from build123d import *

# Parameters (mm, degrees)
ESQUISSE1_W        = 58.2
ESQUISSE1_H        = 40
BOSS_EXTRU_1_DEPTH = 27
ESQUISSE2_R        = 15.5
BOSS_EXTRU_2_DEPTH = 57
ESQUISSE3_R        = 0.796993634
ESQUISSE3_R_2      = 3
ESQUISSE3_R_3      = 2.5
ESQUISSE3_R_4      = 1.643785586
BOSS_EXTRU_3_DEPTH = 1
ESQUISSE4_R        = 0.796993634
ESQUISSE4_R_2      = 3
ESQUISSE4_R_3      = 2.765269511
ESQUISSE4_R_4      = 2.5
ESQUISSE4_R_5      = 2.472480212
ESQUISSE4_R_6      = 1.643785586
BOSS_EXTRU_4_DEPTH = 1
ESQUISSE5_R        = 8.5
BOSS_EXTRU_5_DEPTH = 2
ESQUISSE6_R        = 3.91408695
BOSS_EXTRU_6_DEPTH = 13


with BuildPart() as part:
    # Esquisse1 → Boss.-Extru.1 (new body)
    with BuildSketch(Plane.XY):
        with Locations((-1.276315789, -5.258552632)):
            Rectangle(ESQUISSE1_W, ESQUISSE1_H)
    extrude(amount=BOSS_EXTRU_1_DEPTH)

    # Esquisse2 → Boss.-Extru.2 (add)
    with BuildSketch(Plane(origin=(27.823684211, 0, 0), x_dir=(0, 0, -1), z_dir=(1, 0, 0))):
        with Locations((-15.74475958, -4.690804329)):
            Circle(ESQUISSE2_R)
    extrude(amount=BOSS_EXTRU_2_DEPTH)

    # Esquisse3 → Boss.-Extru.3 (add)
    with BuildSketch(Plane(origin=(0, 0, 0), x_dir=(-1, 0, 0), z_dir=(0, 0, -1))):
        with Locations((28.393888361, 12.845029268)):
            Circle(ESQUISSE3_R)
        with Locations((28.393888361, -23.584885169)):
            Circle(ESQUISSE3_R)
        with Locations((-26.168877972, 12.845029268)):
            Circle(ESQUISSE3_R)
        with Locations((-26.168877972, -23.584885169)):
            Circle(ESQUISSE3_R)
        with Locations((23.719200753, 10.39595939)):
            Circle(ESQUISSE3_R_2)
        with Locations((23.719200753, -20.319458665)):
            Circle(ESQUISSE3_R_2)
        with Locations((-21.69063657, -20.319458665)):
            Circle(ESQUISSE3_R_3)
        with Locations((-5.740000065, -0.085037149)):
            Circle(ESQUISSE3_R_3)
        with Locations((-5.569925768, -9.387416532)):
            Circle(ESQUISSE3_R_3)
        with BuildLine():
            Line((-16.903552301, 11.389352188), (-13.903552301, 7.389352188))
            ThreePointArc((-13.903552301, 7.389352188), (-14.703552301, 1.789352188), (-20.303552301, 2.589352188))
            Line((-20.303552301, 2.589352188), (-23.303552301, 6.589352188))
            ThreePointArc((-23.303552301, 6.589352188), (-22.503552301, 12.189352188), (-16.903552301, 11.389352188))
        make_face()
        with Locations((-20.103552301, 8.989352188)):
            Circle(ESQUISSE3_R_4, mode=Mode.SUBTRACT)
    extrude(amount=BOSS_EXTRU_3_DEPTH)

    # Esquisse4 → Boss.-Extru.4 (add)
    with BuildSketch(Plane.XY.offset(27)):
        with Locations((25.547055264, 13.126910984)):
            Circle(ESQUISSE4_R)
        with Locations((25.547055264, -23.303003453)):
            Circle(ESQUISSE4_R)
        with Locations((-28.053751612, 13.126910984)):
            Circle(ESQUISSE4_R)
        with Locations((-28.053751612, -23.303003453)):
            Circle(ESQUISSE4_R)
        with Locations((6.254872146, -1.609813965)):
            Circle(ESQUISSE4_R_2)
        with Locations((6.671158294, -10.421952213)):
            Circle(ESQUISSE4_R_3)
        with Locations((-24.425601337, 9.932760917)):
            Circle(ESQUISSE4_R_4)
        with Locations((21.931193301, -20.852114314)):
            Circle(ESQUISSE4_R_4)
        with Locations((-24.889302534, -19.715256897)):
            Circle(ESQUISSE4_R_5)
        with BuildLine():
            Line((19.844554955, 9.933092183), (22.844554955, 5.933092183))
            ThreePointArc((22.844554955, 5.933092183), (22.044554955, 0.333092183), (16.444554955, 1.133092183))
            Line((16.444554955, 1.133092183), (13.444554955, 5.133092183))
            ThreePointArc((13.444554955, 5.133092183), (14.244554955, 10.733092183), (19.844554955, 9.933092183))
        make_face()
        with Locations((16.644554955, 7.533092183)):
            Circle(ESQUISSE4_R_6, mode=Mode.SUBTRACT)
    extrude(amount=BOSS_EXTRU_4_DEPTH)

    # Esquisse5 → Boss.-Extru.5 (add)
    with BuildSketch(Plane(origin=(0, 0, 0), x_dir=(-1, 0, 0), z_dir=(0, 0, -1))):
        with Locations((10.376315789, -4.734018324)):
            Circle(ESQUISSE5_R)
    extrude(amount=BOSS_EXTRU_5_DEPTH)

    # Esquisse6 → Boss.-Extru.6 (add)
    with BuildSketch(Plane(origin=(0, 0, 0), x_dir=(-1, 0, 0), z_dir=(0, 0, -1))):
        with Locations((10.361829536, -4.723039304)):
            Circle(ESQUISSE6_R)
    extrude(amount=BOSS_EXTRU_6_DEPTH)


solid = part.part
Input: part model. Units: mm. Frame: model coordinates. A direction names the side the tool comes from. Round coordinates to 2 decimals unless told otherwise and drop trailing zeros. Order: outer loops, then holes, each group sorted by start corner. A loop starts at its lowest first (then second) coordinate and runs counter-clockwise, first axis right, second up.
1. Cut plane D-D, the plane x = -9. Output: boundary loops of the cut face in (y, z).
The answers:
outline: (-25.26, 0) - (-13.12, 0) - (-13.12, -2) - (-8.39, -2) - (-8.39, -13) - (-1.05, -13) - (-1.05, -2) - (3.65, -2) - (3.65, 0) - (14.74, 0) - (14.74, 27) - (-25.26, 27) - close
2. Cut plane A-A, the plane z = 10.5. Output: boundary loops of the cut face in (x, y).
The answers:
outline: (-30.38, -25.26) - (27.82, -25.26) - (27.82, -19.28) - (84.82, -19.28) - (84.82, 9.89) - (27.82, 9.89) - (27.82, 14.74) - (-30.38, 14.74) - close
3. Set-up query: faces 4 (the face through (27.824, -5, 29)), 5 (the face through (21.324, 7.961, 27.493)), 6 (the face through (3.355, 0.666, -0.493)), 7 (the face through (20.09, -19.16, 27.49)). Return all of +Z, -Z, +X, -X, +Y, -Y with unobstructed straight access to the full face (end or side cutting, diameter ignored); none if empty.
The answers:
face 4: +Z, +Y, -Y
face 5: +Z, +X, +Y
face 6: -Z
face 7: +Z
4. Cut plane B-B, the plane x = 5.74. Output: boundary loops of the cut face in (y, z), then the cut area to 3 significant figures.
The answers:
outline: (-25.26, 0) - (-11.88, 0) - (-11.88, -1) - (-6.89, -1) - (-6.89, 0) - (-2.59, 0) - (-2.59, -1) - (2.41, -1) - (2.41, 0) - (14.74, 0) - (14.74, 27) - (1.35, 27) - (1.35, 28) - (-4.57, 28) - (-4.57, 27) - (-7.82, 27) - (-7.82, 28) - (-13.03, 28) - (-13.03, 27) - (-25.26, 27) - close
area: 1,100 mm2
5. Cut plane C-C, the plane z = 24. Output: boundary loops of the cut face in (x, y), then the cut area to 3 significant figures.
The answers:
outline: (-30.38, -25.26) - (27.82, -25.26) - (27.82, -17.81) - (84.82, -17.81) - (84.82, 8.43) - (27.82, 8.43) - (27.82, 14.74) - (-30.38, 14.74) - close
area: 3,820 mm2
6. Mould query, pull axis X, two halves, no side actions, for faces 1 (the face through (7.554, -10.909, -0.493)), 2 (the face through (19, 7, -1)), 3 (the face through (-30.376, -6, 13)). Classes: released by +X, released by -X, zero draft, split by the parting line, or undercut.
The answers:
face 1: undercut
face 2: zero draft
face 3: released by -X
7. Pin query (flat end, axial travel): P1, Ø0.5, axis at x = -28, y = 13, coming from the +Z side; P2, Ø1.6, axis at x = 20, y = 9.5, coming from the -Z side; P3, Ø0.8, axis at x = -28.5, y = 13, coming from the -Z side. Return the tip coordinate at first contact, or that it passes through.
The answers:
P1: stops at z = 28
P2: stops at z = 0
P3: stops at z = -1
8. Material intervals for line 1 (Z direction, x = 4, y = -2); line 2 (Z direction, x = 16.5, y = 8); line 3 (X direction, y = -20, z = 11), sorted ascending.
The answers:
line 1: z = 0 to 28
line 2: z = -1 to 27
line 3: x = -30.38 to 27.82
